Could you check a few things on this model? Use its own coordinates, in mm. Coordinates: 2 decimals unless noted, no trailing zeros. Loops run counter-clockwise (first coordinate to the right, second up) from the corner with the lowest first, then second, coordinate; pieces in that order, holes last. Notation, with made-up numbers: M -37,66.25 L -22,66.25 A25 cw -22,94.25 Z; hole C 76.5,8.5 d11. An arc over 180 degrees is marked long. Write each question's results on one line, items separated by ' | '.
```python
from build123d import *

# Parameters (mm, degrees)
CROQUIS1_W              = 210
CROQUIS1_H              = 210
CROQUIS1_R              = 3.25
SALIENTE_EXTRUIR1_DEPTH = 5
REDONDEO1_R             = 2


with BuildPart() as part:
    # Croquis1 → Saliente-Extruir1 (new body)
    with BuildSketch(Plane.XY):
        Rectangle(CROQUIS1_W, CROQUIS1_H)
        with Locations((-12.5, 12.5)):
            Circle(CROQUIS1_R, mode=Mode.SUBTRACT)
        with Locations((12.5, 12.5)):
            Circle(CROQUIS1_R, mode=Mode.SUBTRACT)
        with Locations((-12.5, -12.5)):
            Circle(CROQUIS1_R, mode=Mode.SUBTRACT)
        with Locations((12.5, -12.5)):
            Circle(CROQUIS1_R, mode=Mode.SUBTRACT)
    extrude(amount=SALIENTE_EXTRUIR1_DEPTH)

    # Redondeo1
    redondeo1_edges = [part.edges().sort_by_distance(p)[0] for p in [
        (-105, 105, 2.5),
        (105, 105, 2.5),
        (105, -105, 2.5),
        (-105, -105, 2.5),
    ]]
    fillet(redondeo1_edges, radius=REDONDEO1_R)


solid = part.part
```
(1) Please list where these lines run through material, in increasing order: probe 1 along Y at (x, z) = (12.5, 3.6); probe 2 along X at (y, z) = (-11, 4.25). Write a range as from..to.
Reported:
probe 1: y = -105..-15.75, -9.25..9.25, 15.75..105 | probe 2: x = -105..-15.38, -9.62..9.62, 15.38..105
(2) If we mould it in two halves opening along X, with no side actions, what happens to faces 1 (the flat face through (-1, -105, 2)), 2 (the cylindrical face through (9.253, 12.643, 2.465)), 3 (the flat face through (105, -1, 2))? For each: released by +X, released by -X, zero draft, split by the parting line, or undercut.
Reported:
face 1: zero draft | face 2: undercut | face 3: released by +X
(3) Imagine slicing it at A-A, the plane y = -12.5. List the corners of the cut face in (x, z) for me.
Reported:
outline: M -105,0 L -15.75,0 L -15.75,5 L -105,5 Z; M -9.25,0 L 9.25,0 L 9.25,5 L -9.25,5 Z; M 15.75,0 L 105,0 L 105,5 L 15.75,5 Z
